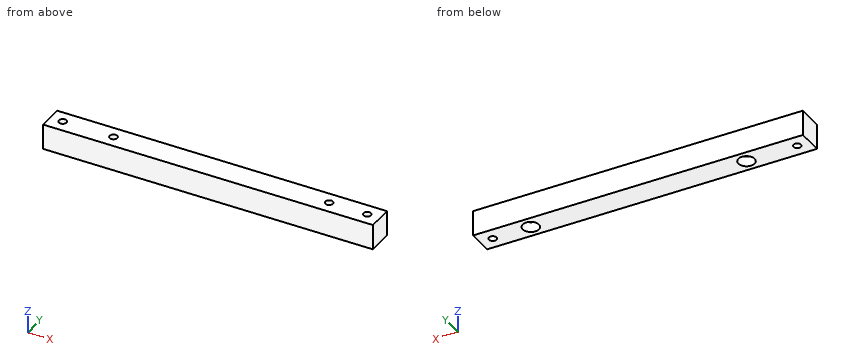
from build123d import *

# Parameters (mm, degrees)
SKETCH_W     = 130
SKETCH_H     = 10
SKETCH_R     = 1.5
PAD_DEPTH    = 10
SKETCH001_R  = 3.2
POCKET_DEPTH = 4


with BuildPart() as part:
    # Sketch → Pad (new body)
    with BuildSketch(Plane.XY):
        with Locations((65, 5)):
            Rectangle(SKETCH_W, SKETCH_H)
        with Locations((5, 5)):
            Circle(SKETCH_R, mode=Mode.SUBTRACT)
        with Locations((25, 5)):
            Circle(SKETCH_R, mode=Mode.SUBTRACT)
        with Locations((125, 5)):
            Circle(SKETCH_R, mode=Mode.SUBTRACT)
        with Locations((110, 5)):
            Circle(SKETCH_R, mode=Mode.SUBTRACT)
    extrude(amount=PAD_DEPTH)

    # Sketch001 (on Face9 of Pad) → Pocket (cut)
    with BuildSketch(Plane(origin=(0, 0, 0), x_dir=(1, 0, 0), z_dir=(0, 0, -1))):
        with Locations((25, -5)):
            Circle(SKETCH001_R)
        with Locations((110, -5)):
            Circle(SKETCH001_R)
    extrude(amount=-POCKET_DEPTH, mode=Mode.SUBTRACT)


solid = part.part
Could you check a few things on this model? Use its own coordinates, in mm. Coordinates: 2 decimals unless noted, no trailing zeros. Order: outer loops, then holes, each group sorted by start corner. A loop starts at its lowest first (then second) coordinate and runs counter-clockwise, first axis right, second up. Notation, with made-up numbers: (-22.75, 38) - (33.25, 38) arc R18 ccw to (33.25, 60) - close; hole circle Ø4 at (-20.75, -37). An arc over 180 degrees is marked (long way). Answer in a Markdown table with one row per item. Add a question column.
(1) If we section it at A-A, the plane z = 5.75: Please give me the cut outline in (x, y), then the cut area to 3 significant figures.
(2) If we section it at B-B, the plane x = 5: Please give me the cut outline in (y, z).
(3) If we section it at C-C, the plane x = 25: Please give me the cut outline in (y, z), then the cut area to 3 significant figures.
(4) Will this pin go through, and if not, where does the flat tip stop? pin 1 (3.5 mm diameter, centred on x = 110, y = 5, fed in from -Z).
(5) I need wall thicknesses on L1, parallel to X at y = 5.5, z = 5.5; L2, parallel to Y at x = 25, z = 1.4; L3, parallel to X at y = 6, z = 5.5. Which ranges of each line are inside material? Lowest first, please.
Results are:
| question | item | result |
|---|---|---|
| 1 | outline | (0, 0) - (130, 0) - (130, 10) - (0, 10) - close; hole circle Ø3 at (5, 5); hole circle Ø3 at (25, 5); hole circle Ø3 at (110, 5); hole circle Ø3 at (125, 5) |
| 1 | area | 1,270 mm2 |
| 2 | outline | (0, 0) - (3.5, 0) - (3.5, 10) - (0, 10) - close; (6.5, 0) - (10, 0) - (10, 10) - (6.5, 10) - close |
| 3 | outline | (0, 0) - (1.8, 0) - (1.8, 4) - (3.5, 4) - (3.5, 10) - (0, 10) - close; (6.5, 4) - (8.2, 4) - (8.2, 0) - (10, 0) - (10, 10) - (6.5, 10) - close |
| 3 | area | 56.4 mm2 |
| 4 | pin 1 | stops at z = 4 |
| 5 | L1 | x = 0 to 3.59, 6.41 to 23.59, 26.41 to 108.59, 111.41 to 123.59, 126.41 to 130 |
| 5 | L2 | y = 0 to 1.8, 8.2 to 10 |
| 5 | L3 | x = 0 to 3.88, 6.12 to 23.88, 26.12 to 108.88, 111.12 to 123.88, 126.12 to 130 |
